Verification items for the finished model (mm, model axes). Face numbers are marked on the shaded views. A direction names the side the tool comes from. Round coordinates to 2 decimals unless told otherwise and drop trailing zeros. Order: outer loops, then holes, each group sorted by start corner. A loop starts at its lowest first (then second) coordinate and runs counter-clockwise, first axis right, second up. Notation, with made-up numbers: M 73,14 L 79,14 A29 cw 79,46 Z; hole C 2.25,13.25 d7. An arc over 180 degrees is marked long. Return JSON: item names as keys, results as strings. Group by question number.
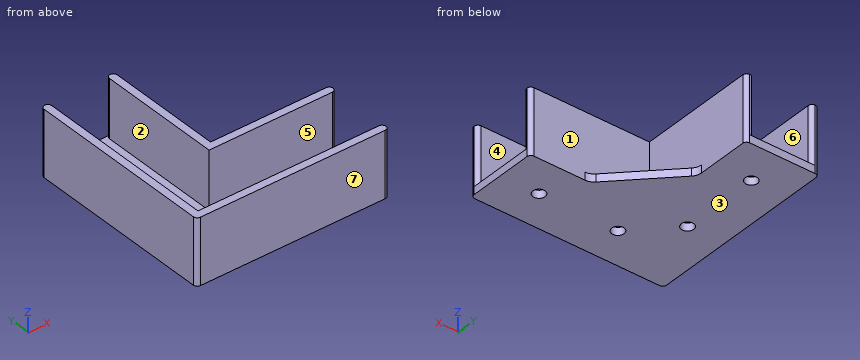
from build123d import *

# Parameters (mm, degrees)
F1_DEPTH = 17
F3_DEPTH = 15
F4_R     = 1.6
F5_DEPTH = 2
F6_R     = 0.99999
F8_DEPTH = 15
F9_R     = 3


# Not quite as in the source:
# - a fillet or chamfer is up to 0.001 mm smaller than in the source, because OpenCascade refuses the exact size


with BuildPart() as f1:
    # F0 (on Top) → F1 (new body)
    with BuildSketch(Plane.XY):
        Polygon((-6, 25), (-25, 25), (-25, -25), (25, -25), (25, -6), (9.5, -6), (-6, -6), (-6, 9.5), align=None)
        Polygon((9.5, -6), (-6, 9.5), (-6, -6), align=None)
    extrude(amount=F1_DEPTH)

    # F2 (on face) → F3 (cut)
    with BuildSketch(Plane.XY.offset(17)):
        Polygon((-8, 25), (-23, 25), (-23, -23), (25, -23), (25, -8), (-6, -8), (-8, -8), (-8, -6), align=None)
    extrude(amount=-F3_DEPTH, mode=Mode.SUBTRACT)

    # F4 (on face) → F5 (cut, through all)
    with BuildSketch(Plane(origin=(0, 0, 0), x_dir=(1, 0, 0), z_dir=(0, 0, -1))):
        with Locations((15, 15.5)):
            Circle(F4_R)
        with Locations((-5.5, 15.5)):
            Circle(F4_R)
        with Locations((-15.5, 5.5)):
            Circle(F4_R)
        with Locations((-15.5, -15)):
            Circle(F4_R)
    extrude(amount=-F5_DEPTH, mode=Mode.SUBTRACT)

    # F6 (radius 1 in the source; OpenCascade refuses exactly that, so slightly less here)
    f6_edges = [f1.edges().sort_by_distance(p)[0] for p in [
        (25, -25, 8.5),
        (25, -23, 9.5),
        (25, -8, 9.5),
        (25, -6, 8.5),
        (-25, -25, 8.5),
        (-25, 25, 8.5),
        (-8, 25, 9.5),
        (-23, 25, 9.5),
        (-6, 25, 8.5),
    ]]
    fillet(f6_edges, radius=F6_R)

    # F7 (on face) → F8 (cut)
    with BuildSketch(Plane.XY.offset(17)):
        Polygon((-6, -6), (9.5, -6), (-6, 9.5), align=None)
    extrude(amount=-F8_DEPTH, mode=Mode.SUBTRACT)

    # F9
    f9_edges = [f1.edges().sort_by_distance(p)[0] for p in [
        (-6, 9.5, 1),
        (9.5, -6, 1),
    ]]
    fillet(f9_edges, radius=F9_R)


solid = f1.part
1. Cross-section at C-C (x = 15). Enter the section's corners in (y, z).
2. Cross-section at A-A (y = -15.5). Enter the section's corners in (x, z), plus the area to 3 significant figures.
3. Go/stop test with flat-tipped pins: pin 1 (3 mm diameter, centred on x = -15.5, y = -5.5, fed in from -Z); pin 2 (12 mm diameter, centred on x = 16.5, y = -19.5, fed in from +Z); pin 3 (8.5 mm diameter, centred on x = 9, z = 7, fed in from +Y); pin 4 (8 mm diameter, centred on x = -14, y = -4, fed in from +Z). Record where each tip stops, or that it passes through.
4. Access from +Z, -Z, +X, -X, +Y, -Y to the whole of each face (thin tool, end or side, straight path). Record for the marked faces 1, 2 and 3.
5. Draft check along Y on the marked faces 4, 5, 6 and 7. Enter one of: +Y half, -Y half, draft (parallel to the pull), parting line (faces both ways), or undercut.
6. Thickness scan on line 1 along Y through (x, z) = (-15.5, 1.65); line 2 along Y through (x, z) = (15, 15). Record the ranges inside material, lowest first. Write a range as from..to.
7. Cross-section at D-D (x = -1). Enter the section's corners in (y, z).
Computed:
{
 "1": {"outline": "M -25,0 L -17.1,0 L -17.1,2 L -23,2 L -23,17 L -25,17 Z; M -13.9,0 L -6,0 L -6,17 L -8,17 L -8,2 L -13.9,2 Z"},
 "2": {"outline": "M -25,0 L -7.1,0 L -7.1,2 L -23,2 L -23,17 L -25,17 Z; M -3.9,0 L 13.4,0 L 13.4,2 L -3.9,2 Z; M 16.6,0 L 25,0 L 25,2 L 16.6,2 Z", "area": "117 mm²"},
 "3": {"pin 1": "passes through", "pin 2": "stops at z = 17", "pin 3": "stops at y = -6", "pin 4": "stops at z = 2"},
 "4": {"face 1": "+Z, +X, +Y", "face 2": "+Z, +Y", "face 3": "-Z, +X, -X, +Y, -Y"},
 "5": {"face 4": "undercut", "face 5": "undercut", "face 6": "draft", "face 7": "-Y half"},
 "6": {"line 1": "y = -25..-7.1, -3.9..13.4, 16.6..25", "line 2": "y = -25..-23, -8..-6"},
 "7": {"outline": "M -25,0 L 4.5,0 L 4.5,2 L -6,2 L -6,17 L -8,17 L -8,2 L -23,2 L -23,17 L -25,17 Z"}
}
